For this review, take the finished solid that the model builds, in its own axes (mm). Round coordinates to 2 decimals unless told otherwise and drop trailing zeros. Order: outer loops, then holes, each group sorted by start corner. A loop starts at its lowest first (then second) coordinate and runs counter-clockwise, first axis right, second up. Notation, with made-up numbers: M 55.25,89 L 73.25,89 A21 ccw 73.25,110 Z; hole C -40,-10.5 d6. An arc over 180 degrees is marked long. Put each result on its own line as item: value.
from build123d import *

# Parameters (mm, degrees)
SKETCH1_W           = 130
SKETCH1_H           = 60
SKETCH1_R           = 4.499999999
BOSS_EXTRUDE1_DEPTH = 10


with BuildPart() as part:
    # Sketch1 → Boss-Extrude1 (new body)
    with BuildSketch(Plane(origin=(0, 0, 0), x_dir=(0, 0, -1), z_dir=(1, 0, 0))):
        with Locations((3.813160791, 27.897530874)):
            Rectangle(SKETCH1_W, SKETCH1_H)
        with Locations((3.813160791, 27.897530874)):
            Circle(SKETCH1_R, mode=Mode.SUBTRACT)
        with BuildLine():
            Line((-5.464379102, 30.775341326), (-4.081605515, 33.606305024))
            ThreePointArc((-4.081605515, 33.606305024), (-1.369183898, 34.499769949), (-0.528409533, 31.770555947))
            Line((-0.528409533, 31.770555947), (-1.869576404, 29.020756356))
            ThreePointArc((-1.869576404, 29.020756356), (-4.544523089, 28.10012945), (-5.464379102, 30.775341326))
        make_face(mode=Mode.SUBTRACT)
        with BuildLine():
            Line((5.31316079, 18.397530874), (2.313160791, 18.397530874))
            ThreePointArc((2.313160791, 18.397530874), (0.313160792, 20.397530874), (2.313160791, 22.397530873))
            Line((2.313160791, 22.397530873), (5.31316079, 22.397530873))
            ThreePointArc((5.31316079, 22.397530873), (7.313160789, 20.397530874), (5.31316079, 18.397530874))
        make_face(mode=Mode.SUBTRACT)
        with BuildLine():
            Line((5.31316079, 33.374248764), (2.313160791, 33.374248764))
            ThreePointArc((2.313160791, 33.374248764), (0.31316079, 35.374248765), (2.313160791, 37.374248765))
            Line((2.313160791, 37.374248765), (5.31316079, 37.374248765))
            ThreePointArc((5.31316079, 37.374248765), (7.313160791, 35.374248765), (5.31316079, 33.374248764))
        make_face(mode=Mode.SUBTRACT)
        with BuildLine():
            Line((9.471997672, 29.038205562), (8.081045524, 31.961596177))
            ThreePointArc((8.081045524, 31.961596177), (9.113942414, 34.555839775), (11.733632625, 33.589300054))
            Line((11.733632625, 33.589300054), (13.083423708, 30.758314735))
            ThreePointArc((13.083423708, 30.758314735), (12.137765277, 28.092547131), (9.471997672, 29.038205562))
        make_face(mode=Mode.SUBTRACT)
    extrude(amount=BOSS_EXTRUDE1_DEPTH)


solid = part.part
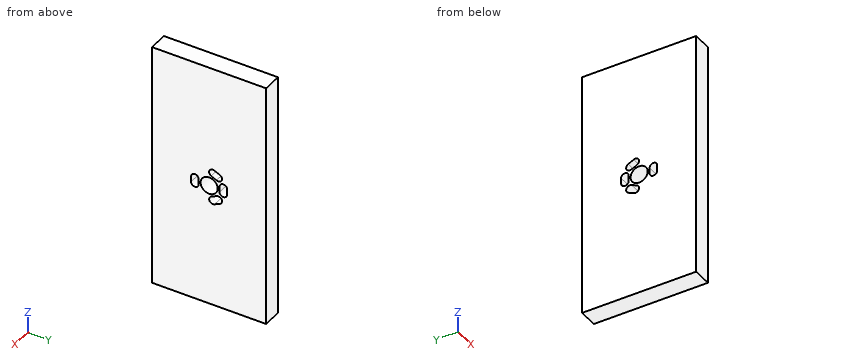
(1) Add section A-A on y = 26. Give the boundary of the cut face in (x, z).
A:
outline: M 0,-68.81 L 10,-68.81 L 10,-7.89 L 0,-7.89 Z; M 0,0.27 L 10,0.27 L 10,61.19 L 0,61.19 Z
(2) To check wall thickness, follow L1, parallel to Z at x = 5.5, y = 30; L2, parallel to Z at x = 4.5, y = 34; L3, parallel to Z at x = 4.5, y = 33. State the ranges of each line that lie inside material, in increasing order.
A:
L1: z = -68.81 to -13.28, -9.01 to -7.79, 0.17 to 1.39, 5.66 to 61.19
L2: z = -68.81 to -11.47, -8.38 to -6.77, -0.86 to 0.75, 3.83 to 61.19
L3: z = -68.81 to -12.01, -7.95 to 0.31, 4.38 to 61.19
(3) Add section B-B on x = 5.5. Give the boundary of the cut face in (y, z), then the cut area to 3 significant figures.
A:
outline: M -2.1,-68.81 L 57.9,-68.81 L 57.9,61.19 L -2.1,61.19 Z; hole M 18.4,-5.31 A2 ccw 22.4,-5.31 L 22.4,-2.31 A2 ccw 18.4,-2.31 Z; hole C 27.9,-3.81 d9; hole M 29.02,1.87 L 31.77,0.53 A2 ccw long 33.61,4.08 L 30.78,5.46 A2 ccw Z; hole M 29.04,-9.47 A2 ccw 30.76,-13.08 L 33.59,-11.73 A2 ccw 31.96,-8.08 Z; hole M 33.37,-5.31 A2 ccw 37.37,-5.31 L 37.37,-2.31 A2 ccw 33.37,-2.31 Z
area: 7,640 mm2
